The drawing under review shows one solid part. Ordinate dimensions are in mm from its lowest x, y, z. A direction names the side the tool comes from. Round coordinates to 2 decimals unless told otherwise and drop trailing zeros. Write each loop counter-clockwise with the first axis right and the second up, starting at its lowest first coordinate (ties: lowest second). Pieces come first, ordered by that corner, then holes. Notation, with made-up numbers: (33, 71) -> (85, 71) arc R24 ccw to (85, 106) -> close; hole circle Ø7 at (-7, -0.5). An arc over 180 degrees is marked (long way). Write item = value, one per line. Start each with the question number.
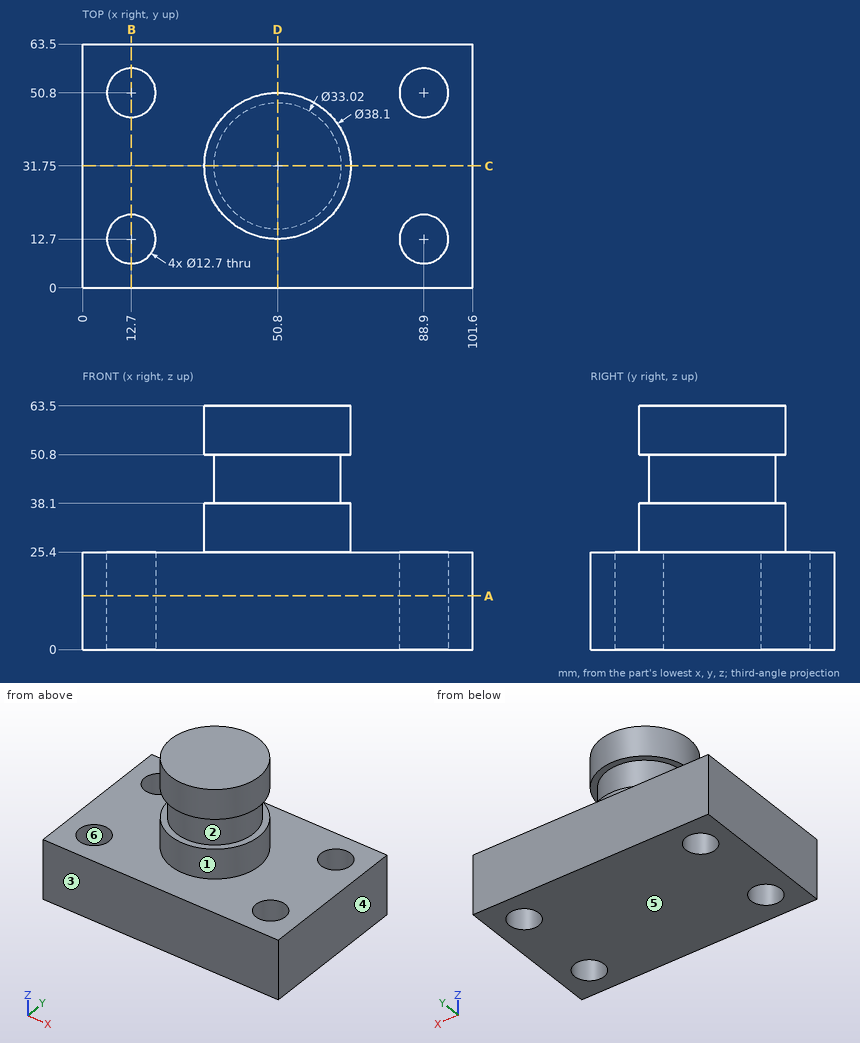
1. Clearance check with flat-ended pins moving along their axes: pin 1 Ø5 at (x, y) = (62, 14) entering from -Z; pin 2 Ø12 at (x, y) = (83, 43) entering from +Z; pin 3 Ø5 at (x, z) = (70, 46.5) entering from -Y; pin 4 Ø5 at (y, z) = (36, 48.5) entering from -X. State where each tip first meets the part, or that it passes through.
2. Consider section D-D, the plane x = 50.8. Give the boundary of the cut face in (y, z), then the cut area to 3 significant figures.
3. Machinability: for the marked faces 1, 2 and 3, which of the approach directions +Z, -Z, +X, -X, +Y, -Y give a long, thin tool a straight path to every point of the face, cutting with its end or side? Answer none if there is none.
4. Consider section C-C, the plane y = 31.75. Give the boundary of the cut face in (x, z), then the cut area to 3 significant figures.
5. Draft analysis for pull direction X (two halves, no side actions). For the marked faces 4, 5 and 6, state which applies: +X half, -X half, draft (parallel to the pull), parting line (faces both ways), or undercut.
6. Wall thickness on L1, parallel to Y at x = 88.9, z = 14.5; L2, parallel to X at y = 17, z = 14; L3, parallel to X at y = 50, z = 8: over which ranges is each line inside the solid? List them lowest first. Write a range as from..to.
7. Consider section B-B, the plane x = 12.7. Give the boundary of the cut face in (y, z), then the cut area to 3 significant figures.
8. Consider section A-A, the plane z = 14. Give the boundary of the cut face in (x, y), then the cut area to 3 significant figures.
Outcome:
q1.pin_1 = 0
q1.pin_2 = 25.4
q1.pin_3 = through
q1.pin_4 = 32.03
q2.outline = (0, 0) -> (63.5, 0) -> (63.5, 25.4) -> (50.8, 25.4) -> (50.8, 38.1) -> (48.26, 38.1) -> (48.26, 50.8) -> (50.8, 50.8) -> (50.8, 63.5) -> (12.7, 63.5) -> (12.7, 50.8) -> (15.24, 50.8) -> (15.24, 38.1) -> (12.7, 38.1) -> (12.7, 25.4) -> (0, 25.4) -> close
q2.area = 3,000 mm2
q3.face_1 = +Z
q3.face_2 = none
q3.face_3 = +Z, -Z, +X, -X, -Y
q4.outline = (0, 0) -> (101.6, 0) -> (101.6, 25.4) -> (69.85, 25.4) -> (69.85, 38.1) -> (67.31, 38.1) -> (67.31, 50.8) -> (69.85, 50.8) -> (69.85, 63.5) -> (31.75, 63.5) -> (31.75, 50.8) -> (34.29, 50.8) -> (34.29, 38.1) -> (31.75, 38.1) -> (31.75, 25.4) -> (0, 25.4) -> close
q4.area = 3,970 mm2
q5.face_4 = +X half
q5.face_5 = draft
q5.face_6 = undercut
q6.L1 = 0..6.35, 19.05..44.45, 57.15..63.5
q6.L2 = 0..8.03, 17.37..84.23, 93.57..101.6
q6.L3 = 0..6.4, 19..82.6, 95.2..101.6
q7.outline = (0, 0) -> (6.35, 0) -> (6.35, 25.4) -> (0, 25.4) -> close; (19.05, 0) -> (44.45, 0) -> (44.45, 25.4) -> (19.05, 25.4) -> close; (57.15, 0) -> (63.5, 0) -> (63.5, 25.4) -> (57.15, 25.4) -> close
q7.area = 968 mm2
q8.outline = (0, 0) -> (101.6, 0) -> (101.6, 63.5) -> (0, 63.5) -> close; hole circle Ø12.7 at (12.7, 12.7); hole circle Ø12.7 at (12.7, 50.8); hole circle Ø12.7 at (88.9, 12.7); hole circle Ø12.7 at (88.9, 50.8)
q8.area = 5,940 mm2
